Part model, mm, in its own coordinate system. Face numbers are marked on the shaded views. A direction names the side the tool comes from. Give positions to 0.01 mm unless a question says otherwise; leave off trailing zeros. Order: outer loops, then holes, each group sorted by start corner. A loop starts at its lowest first (then second) coordinate and runs counter-clockwise, first axis right, second up. Notation, with made-up numbers: M 11.5,-19 L 48.5,-19 A37 cw 48.5,18 Z; hole C 13.5,12.5 d3. An arc over 180 degrees is marked long. Answer as a JSON object with one key per item and string values.
from build123d import *

# Parameters (mm, degrees)
F0_W     = 25.4
F0_H     = 12.7
F0_H_2   = 31.75
F1_DEPTH = 25.4
F2_R     = 6.35
F3_DEPTH = 25.4
F4_R     = 6.35
F5_DEPTH = 25.4
F7_DEPTH = 25.4


with BuildPart() as f1:
    # F0 (on Front) → F1 (new body)
    with BuildSketch(Plane.XZ):
        with Locations((12.7, 6.35)):
            Rectangle(F0_W, F0_H)
        with Locations((38.1, 6.35)):
            Rectangle(F0_W, F0_H)
        with Locations((63.5, 6.35)):
            Rectangle(F0_W, F0_H)
        with Locations((38.1, 28.575)):
            Rectangle(F0_W, F0_H_2)
    extrude(amount=F1_DEPTH)

    # F2 (on face) → F3 (cut)
    with BuildSketch(Plane(origin=(25.4, 0, 0), x_dir=(0, -1, 0), z_dir=(-1, 0, 0))):
        with Locations((12.7, 31.75)):
            Circle(F2_R)
        with BuildLine():
            ThreePointArc((0, 32.2180166472), (2.9688610836, 40.1479347861), (10.2620066819, 44.45))
            Line((10.2620066819, 44.45), (0, 44.45))
            Line((0, 44.45), (0, 32.2180166472))
        make_face()
        with BuildLine():
            ThreePointArc((15.1379933181, 44.45), (22.4311389164, 40.1479347861), (25.4, 32.2180166472))
            Line((25.4, 32.2180166472), (25.4, 44.45))
            Line((25.4, 44.45), (15.1379933181, 44.45))
        make_face()
    extrude(amount=-F3_DEPTH, mode=Mode.SUBTRACT)

    # F4 (on face) → F5 (cut)
    with BuildSketch(Plane.XY.offset(12.7)):
        with Locations((12.7, -12.7)):
            Circle(F4_R)
        with Locations((63.5, -12.7)):
            Circle(F4_R)
        with BuildLine():
            ThreePointArc((0, -12.7), (3.7197438789, -3.7197438789), (12.7, 0))
            Line((12.7, 0), (0, 0))
            Line((0, 0), (0, -12.7))
        make_face()
        with BuildLine():
            ThreePointArc((12.7, -25.4), (3.7197438789, -21.6802561211), (0, -12.7))
            Line((0, -12.7), (0, -25.4))
            Line((0, -25.4), (12.7, -25.4))
        make_face()
    extrude(amount=-F5_DEPTH, mode=Mode.SUBTRACT)

    # F6 (on face) → F7 (cut)
    with BuildSketch(Plane.XY.offset(12.7)):
        with BuildLine():
            ThreePointArc((63.5, 0), (76.1234988118, -12.7), (63.5, -25.4))
            Line((63.5, -25.4), (76.2, -25.4))
            Line((76.2, -25.4), (76.2, 0))
            Line((76.2, 0), (63.5, 0))
        make_face()
    extrude(amount=-F7_DEPTH, mode=Mode.SUBTRACT)


solid = f1.part
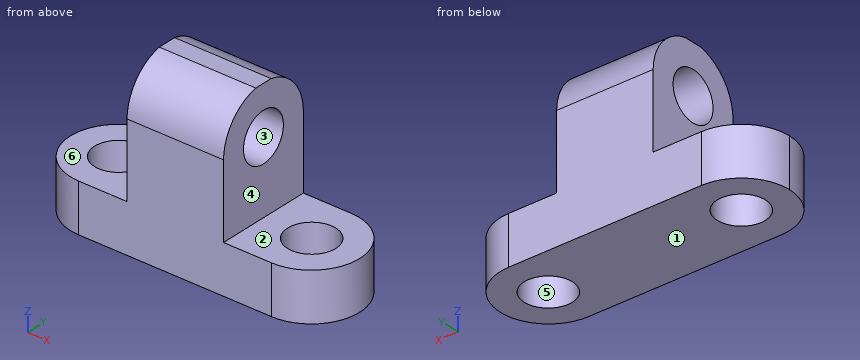
1. Cut at B-B on z = 6.5. Give the cut face in (x, y), plus the area to 3 significant figures.
Worked answers:
{"outline": "M 12.7,-25.4 L 63.5,-25.4 A12.7 ccw 63.5,0 L 12.7,0 A12.7 ccw Z; hole C 12.7,-12.7 d12.7; hole C 63.5,-12.7 d12.7", "area": "1,540 mm^2"}
2. Cut at A-A on x = 29. Give the cut face in (y, z), plus the area to 3 significant figures.
Worked answers:
{"outline": "M -25.4,0 L 0,0 L 0,32.22 A12.7 ccw -10.26,44.45 L -15.14,44.45 A12.7 ccw -25.4,32.22 Z; hole C -12.7,31.75 d12.7", "area": "938 mm^2"}
3. Pin check, flat tips, straight feed: P1, Ø1.5, axis at y = -4.5, z = 15.5, coming from the +X side; P2, Ø7.5, axis at x = 12, y = -18, coming from the +Z side; P3, Ø5, axis at y = -20, z = 14.5, coming from the +X side. Stop position of each tip, or through.
Worked answers:
{"P1": "stops at x = 50.8", "P2": "stops at z = 12.7", "P3": "stops at x = 74.84"}
4. Which spindle directions (+Z, -Z, +X, -X, +Y, -Y) get a long thin tool onto all of the face, cutting with end or side? Do the marked faces 5 and 6. Say none if no direction does.
Worked answers:
{"face 5": "+Z, -Z", "face 6": "+Z, -X, +Y, -Y"}
5. Cut at C-C on y = -13.5. Give the cut face in (x, z), plus the area to 3 significant figures.
Worked answers:
{"outline": "M 0.03,0 L 6.4,0 L 6.4,12.7 L 0.03,12.7 Z; M 19,0 L 57.2,0 L 57.2,12.7 L 50.8,12.7 L 50.8,25.45 L 25.4,25.45 L 25.4,12.7 L 19,12.7 Z; M 25.4,38.05 L 50.8,38.05 L 50.8,44.45 L 25.4,44.45 Z; M 69.8,0 L 76.1,0 L 76.1,12.7 L 69.8,12.7 Z", "area": "1,130 mm^2"}
6. Two-plate mould, pull along Z, no slides. Class the marked faces 1, 2, 3 and 4: +Z half, -Z half, draft (parallel to the pull), parting line (faces both ways), or undercut.
Worked answers:
{"face 1": "-Z half", "face 2": "+Z half", "face 3": "undercut", "face 4": "draft"}
7. Cut at D-D on x = 17. Give the cut face in (y, z).
Worked answers:
{"outline": "M -25.4,0 L -17.37,0 L -17.37,12.7 L -25.4,12.7 Z; M -8.03,0 L 0,0 L 0,12.7 L -8.03,12.7 Z"}
8. Probe line 1 along X through (y, z) = (-10.5, 3.5); line 2 along Y through (x, z) = (12.7, 10); line 3 along Z through (x, y) = (70, -12.5). List the from-to ranges inside material, lowest first.
Worked answers:
{"line 1": "x = 0.19 to 6.74, 18.66 to 57.54, 69.46 to 75.93", "line 2": "y = -25.4 to -19.05, -6.35 to 0", "line 3": "z = 0 to 12.7"}
